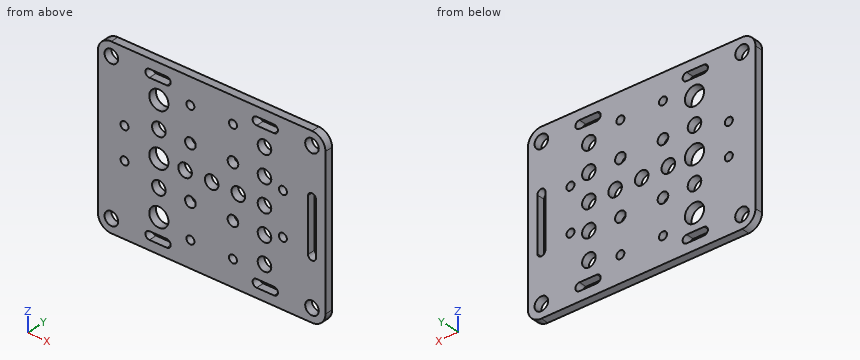
from build123d import *

# Parameters (mm, degrees)
SKETCH1_R           = 2.55
SKETCH1_R_2         = 1.5
SKETCH1_R_3         = 2
SKETCH1_R_4         = 3.6
BOSS_EXTRUDE1_DEPTH = 3


with BuildPart() as part:
    # Sketch1 → Boss-Extrude1 (new body)
    with BuildSketch(Plane(origin=(0, 0, 0), x_dir=(1, 0, 0), z_dir=(0, 1, 0))):
        with BuildLine():
            Line((27.75, -32.75), (-27.75, -32.75))
            Line((-27.75, -32.75), (-37.75, -32.75))
            ThreePointArc((-37.75, -32.75), (-41.285533906, -31.285533906), (-42.75, -27.75))
            Line((-42.75, -27.75), (-42.75, 27.75))
            ThreePointArc((-42.75, 27.75), (-41.285533906, 31.285533906), (-37.75, 32.75))
            Line((-37.75, 32.75), (-27.75, 32.75))
            Line((-27.75, 32.75), (27.75, 32.75))
            Line((27.75, 32.75), (37.75, 32.75))
            ThreePointArc((37.75, 32.75), (41.285533906, 31.285533906), (42.75, 27.75))
            Line((42.75, 27.75), (42.75, -27.75))
            ThreePointArc((42.75, -27.75), (41.285533906, -31.285533906), (37.75, -32.75))
            Line((37.75, -32.75), (27.75, -32.75))
        make_face()
        with Locations((37.7, 27.7)):
            Circle(SKETCH1_R, mode=Mode.SUBTRACT)
        with Locations((37.7, -27.7)):
            Circle(SKETCH1_R, mode=Mode.SUBTRACT)
        with Locations((-37.7, -27.7)):
            Circle(SKETCH1_R, mode=Mode.SUBTRACT)
        with Locations((-37.7, 27.7)):
            Circle(SKETCH1_R, mode=Mode.SUBTRACT)
        with Locations((-8, 23)):
            Circle(SKETCH1_R_2, mode=Mode.SUBTRACT)
        with Locations((-8, 10)):
            Circle(SKETCH1_R_3, mode=Mode.SUBTRACT)
        Circle(SKETCH1_R, mode=Mode.SUBTRACT)
        with Locations((10, 0)):
            Circle(SKETCH1_R, mode=Mode.SUBTRACT)
        with Locations((-10, 0)):
            Circle(SKETCH1_R, mode=Mode.SUBTRACT)
        with Locations((-19.85, 20)):
            Circle(SKETCH1_R_4, mode=Mode.SUBTRACT)
        with Locations((-19.85, 0)):
            Circle(SKETCH1_R_4, mode=Mode.SUBTRACT)
        with Locations((-19.85, -20)):
            Circle(SKETCH1_R_4, mode=Mode.SUBTRACT)
        with Locations((8, 23)):
            Circle(SKETCH1_R_2, mode=Mode.SUBTRACT)
        with Locations((-8, -10)):
            Circle(SKETCH1_R_3, mode=Mode.SUBTRACT)
        with Locations((8, -10)):
            Circle(SKETCH1_R_3, mode=Mode.SUBTRACT)
        with Locations((8, 10)):
            Circle(SKETCH1_R_3, mode=Mode.SUBTRACT)
        with Locations((-19.85, 10)):
            Circle(SKETCH1_R, mode=Mode.SUBTRACT)
        with Locations((-8, -23)):
            Circle(SKETCH1_R_2, mode=Mode.SUBTRACT)
        with Locations((8, -23)):
            Circle(SKETCH1_R_2, mode=Mode.SUBTRACT)
        with Locations((-32.75, 6)):
            Circle(SKETCH1_R_2, mode=Mode.SUBTRACT)
        with Locations((19.85, 20)):
            Circle(SKETCH1_R, mode=Mode.SUBTRACT)
        with Locations((19.85, 0)):
            Circle(SKETCH1_R, mode=Mode.SUBTRACT)
        with Locations((19.85, -20)):
            Circle(SKETCH1_R, mode=Mode.SUBTRACT)
        with Locations((-32.75, -6)):
            Circle(SKETCH1_R_2, mode=Mode.SUBTRACT)
        with Locations((26.75, 8)):
            Circle(SKETCH1_R_2, mode=Mode.SUBTRACT)
        with Locations((26.766687539, -7.999991298)):
            Circle(SKETCH1_R_2, mode=Mode.SUBTRACT)
        with Locations((19.85, 10)):
            Circle(SKETCH1_R, mode=Mode.SUBTRACT)
        with Locations((19.85, -10)):
            Circle(SKETCH1_R, mode=Mode.SUBTRACT)
        with Locations((-19.85, -10)):
            Circle(SKETCH1_R, mode=Mode.SUBTRACT)
        with BuildLine():
            Line((39.2, 10), (39.2, -10))
            ThreePointArc((39.2, -10), (37.7, -11.5), (36.2, -10))
            Line((36.2, -10), (36.2, 10))
            ThreePointArc((36.2, 10), (37.7, 11.5), (39.2, 10))
        make_face(mode=Mode.SUBTRACT)
        with BuildLine():
            Line((-16.9, 26.2), (-23.4, 26.2))
            ThreePointArc((-23.4, 26.2), (-24.9, 27.7), (-23.4, 29.2))
            Line((-23.4, 29.2), (-16.9, 29.2))
            ThreePointArc((-16.9, 29.2), (-15.4, 27.7), (-16.9, 26.2))
        make_face(mode=Mode.SUBTRACT)
        with BuildLine():
            Line((16.9, 26.2), (23.4, 26.2))
            ThreePointArc((23.4, 26.2), (24.9, 27.7), (23.4, 29.2))
            Line((23.4, 29.2), (16.9, 29.2))
            ThreePointArc((16.9, 29.2), (15.4, 27.7), (16.9, 26.2))
        make_face(mode=Mode.SUBTRACT)
        with BuildLine():
            Line((-16.9, -26.2), (-23.4, -26.2))
            ThreePointArc((-23.4, -26.2), (-24.9, -27.7), (-23.4, -29.2))
            Line((-23.4, -29.2), (-16.9, -29.2))
            ThreePointArc((-16.9, -29.2), (-15.4, -27.7), (-16.9, -26.2))
        make_face(mode=Mode.SUBTRACT)
        with BuildLine():
            Line((16.9, -26.2), (23.4, -26.2))
            ThreePointArc((23.4, -26.2), (24.9, -27.7), (23.4, -29.2))
            Line((23.4, -29.2), (16.9, -29.2))
            ThreePointArc((16.9, -29.2), (15.4, -27.7), (16.9, -26.2))
        make_face(mode=Mode.SUBTRACT)
    extrude(amount=BOSS_EXTRUDE1_DEPTH)


solid = part.part
Check sheet for the modelled part. Datum: model origin and axes. Units: mm. Round coordinates to 2 decimals unless told otherwise and drop trailing zeros. Write each loop counter-clockwise with the first axis right and the second up, starting at its lowest first coordinate (ties: lowest second). Pieces come first, ordered by that corner, then holes. Notation, with made-up numbers: (74, 77) -> (80, 77) arc R14 cw to (80, 81) -> close; hole circle Ø8 at (30.25, 34.25). An arc over 180 degrees is marked (long way). Answer as CSV lines item,"result". Start each with the question number.
1) Section check A-A on x = 0. Enter the section's corners in (y, z), and give its area (3 significant figures).
2) Material ranges on line 1 (X direction, y = 2, z = -10); line 2 (X direction, y = 2.3, z = -27.7); line 3 (X direction, y = 1.2, z = -6), recorded low to high. Write a range as from..to.
3) Go/stop test with a flat-tipped pin: P1, Ø1.5, axis at x = -2.5, z = -22, coming from the -Y side. Record where the tip stops, or that it passes through.
4) Section check B-B on z = 20. Enter the section's corners in (x, y).
5) Section check D-D on x = 26.75. Enter the section's corners in (y, z).
6) Section check C-C on z = 0. Enter the section's corners in (x, y), and give its area (3 significant figures).
Found:
1,outline,"(0, -32.75) -> (3, -32.75) -> (3, -2.55) -> (0, -2.55) -> close; (0, 2.55) -> (3, 2.55) -> (3, 32.75) -> (0, 32.75) -> close"
1,area,"181 mm^2"
2,line 1,"x = -42.75..-22.4, -17.3..-10, -6..6, 10..17.3, 22.4..36.2, 39.2..42.75"
2,line 2,"x = -42.75..-40.25, -35.15..-24.9, -15.4..15.4, 24.9..35.15, 40.25..42.75"
2,line 3,"x = -42.75..-34.25, -31.25..36.2, 39.2..42.75"
3,P1,"stops at y = 0"
4,outline,"(-42.75, 0) -> (-23.45, 0) -> (-23.45, 3) -> (-42.75, 3) -> close; (-16.25, 0) -> (17.3, 0) -> (17.3, 3) -> (-16.25, 3) -> close; (22.4, 0) -> (42.75, 0) -> (42.75, 3) -> (22.4, 3) -> close"
5,outline,"(0, -32.75) -> (3, -32.75) -> (3, -9.5) -> (0, -9.5) -> close; (0, -6.5) -> (3, -6.5) -> (3, 6.5) -> (0, 6.5) -> close; (0, 9.5) -> (3, 9.5) -> (3, 32.75) -> (0, 32.75) -> close"
6,outline,"(-42.75, 0) -> (-23.45, 0) -> (-23.45, 3) -> (-42.75, 3) -> close; (-16.25, 0) -> (-12.55, 0) -> (-12.55, 3) -> (-16.25, 3) -> close; (-7.45, 0) -> (-2.55, 0) -> (-2.55, 3) -> (-7.45, 3) -> close; (2.55, 0) -> (7.45, 0) -> (7.45, 3) -> (2.55, 3) -> close; (12.55, 0) -> (17.3, 0) -> (17.3, 3) -> (12.55, 3) -> close; (22.4, 0) -> (36.2, 0) -> (36.2, 3) -> (22.4, 3) -> close; (39.2, 0) -> (42.75, 0) -> (42.75, 3) -> (39.2, 3) -> close"
6,area,"165 mm^2"
